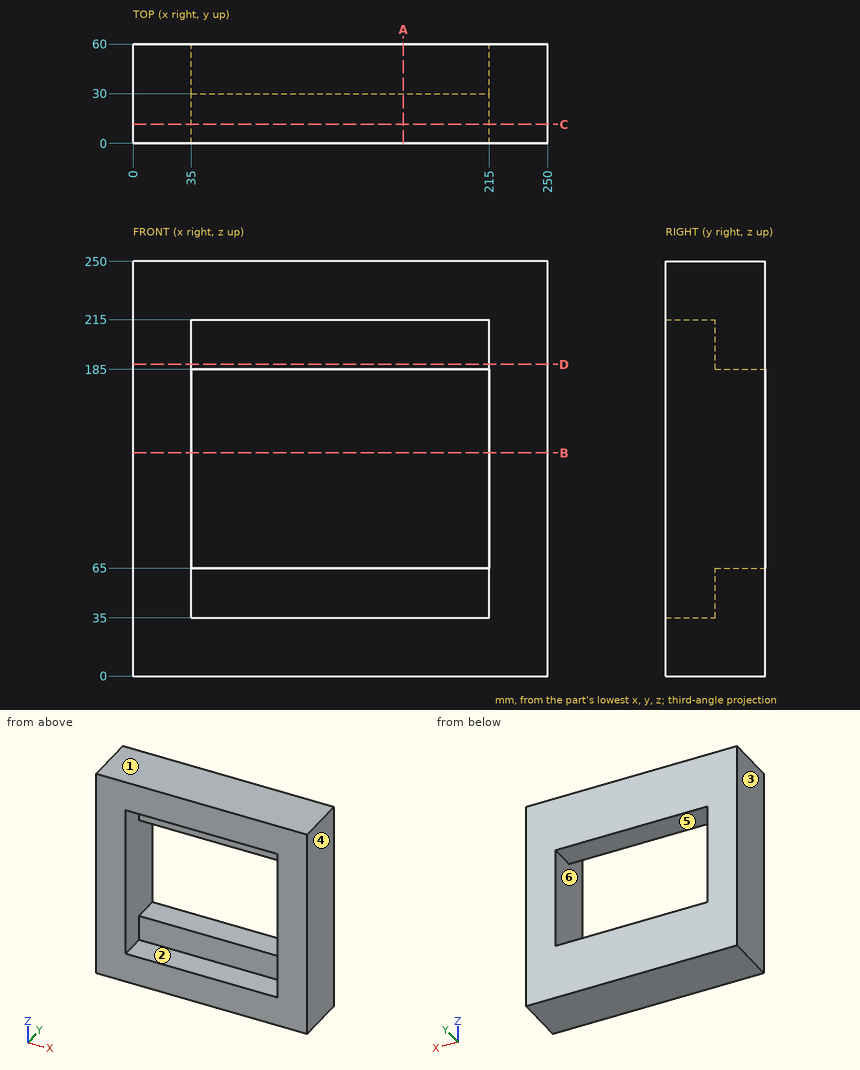
Geometry check sheet. Reference: drawing and pictorial views, mm from the part's lowest x, y, z. A direction names the side the tool comes from. Give positions to 0.01 mm unless a question says otherwise; leave off trailing zeros. Loops run counter-clockwise (first coordinate to the right, second up) from the corner with the lowest first, then second, coordinate; pieces in that order, holes last.
1. Mould release check, pull along Z, two halves, no side actions. Record for the marked faces 1, 2 and 3: released by +Z, released by -Z, zero draft, split by the parting line, or undercut.
2. Thickness scan on line 1 (X direction, y = 32, z = 80.5); line 2 (Z direction, x = 55.5, y = 41). Record the ranges inside material, lowest first.
3. Section check D-D, the plane z = 188. Enter the section's corners in (x, y), then the cut area to 3 significant figures.
4. Set-up check for the marked faces 4, 5 and 6: record each of +Z, -Z, +X, -X, +Y, -Y from which the full face is reachable in a straight line by a thin tool's end or side.
5. Section check C-C, the plane y = 11.5. Enter the section's corners in (x, z), then the cut area to 3 significant figures.
6. Go/stop test with a flat-tipped pin: pin 1 Ø9 at (x, z) = (116.5, 57) entering from -Y. Record where the tip stops, or that it passes through.
7. Section check A-A, the plane x = 163. Enter the section's corners in (y, z), then the cut area to 3 significant figures.
8. Section check B-B, the plane z = 134.5. Enter the section's corners in (x, y).
Geometry says:
1. face 1: released by +Z
1. face 2: undercut
1. face 3: zero draft
2. line 1: x = 0 to 35, 215 to 250
2. line 2: z = 0 to 65, 185 to 250
3. outline: (0, 0) - (35, 0) - (35, 30) - (215, 30) - (215, 0) - (250, 0) - (250, 60) - (0, 60) - close
3. area: 9,600 mm2
4. face 4: +Z, -Z, +X, +Y, -Y
4. face 5: +Y, -Y
4. face 6: -Y
5. outline: (0, 0) - (250, 0) - (250, 250) - (0, 250) - close; hole (35, 35) - (215, 35) - (215, 215) - (35, 215) - close
5. area: 30,100 mm2
6. pin 1: stops at y = 30
7. outline: (0, 0) - (60, 0) - (60, 65) - (30, 65) - (30, 35) - (0, 35) - close; (0, 215) - (30, 215) - (30, 185) - (60, 185) - (60, 250) - (0, 250) - close
7. area: 6,000 mm2
8. outline: (0, 0) - (35, 0) - (35, 60) - (0, 60) - close; (215, 0) - (250, 0) - (250, 60) - (215, 60) - close
